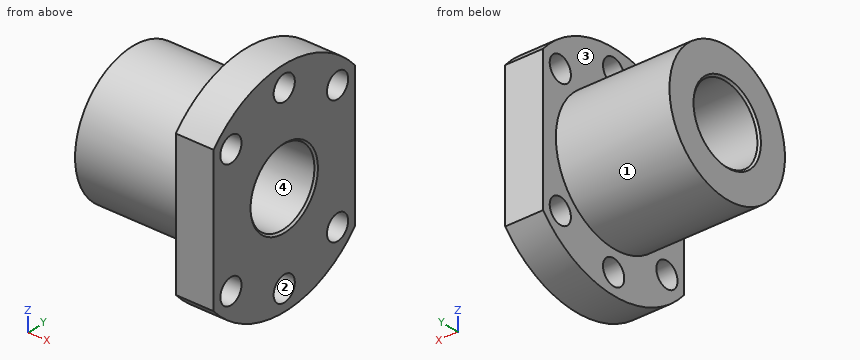
from build123d import *

# Parameters (mm, degrees)
F0_R     = 18
F1_DEPTH = 30
F3_DEPTH = 10
F4_R     = 10
F5_DEPTH = 40.001
F6_SIZE  = 0.5
F8_D     = 6.6


with BuildPart() as f1:
    # F0 (on Right) → F1 (new body)
    with BuildSketch(Plane.YZ):
        Circle(F0_R)
    extrude(amount=-F1_DEPTH)

    # F2 (on face) → F3 (join)
    with BuildSketch(Plane.YZ):
        with BuildLine():
            Line((-22, 18.8944436277), (-22, -18.8944436277))
            ThreePointArc((-22, -18.8944436277), (0, -29), (22, -18.8944436277))
            Line((22, -18.8944436277), (22, 18.8944436277))
            ThreePointArc((22, 18.8944436277), (0, 29), (-22, 18.8944436277))
        make_face()
    extrude(amount=F3_DEPTH)

    # F4 (on face) → F5 (cut, through all)
    with BuildSketch(Plane.YZ.offset(10)):
        Circle(F4_R)
    extrude(amount=-F5_DEPTH, mode=Mode.SUBTRACT)

    # F6
    f6_edges = [f1.edges().sort_by_distance(p)[0] for p in [
        (10, -10, 0),
        (-30, -10, 0),
    ]]
    chamfer(f6_edges, length=F6_SIZE)

    # F8 (through all)
    with Locations(Plane.YZ.offset(10)):
        with Locations((0, 23.5), (16.617, 16.617), (16.617, -16.617), (0, -23.5), (-16.617, -16.617), (-16.617, 16.617)):
            Hole(F8_D / 2)


solid = f1.part
Verification items for the finished model (mm, model axes). Face numbers are marked on the shaded views. Coordinates: 2 decimals unless noted, no trailing zeros. Write each loop counter-clockwise with the first axis right and the second up, starting at its lowest first coordinate (ties: lowest second). Pieces come first, ordered by that corner, then holes. Notation, with made-up numbers: M -35.75,67 L 19.25,67 A34 cw 19.25,100 Z; hole C -31,13.25 d1. An arc over 180 degrees is marked long. Use a Markdown table: item, result.
Q1. Sectioned sample at C-C, the plane x = -17.5. Record the boundary of the cut face in (y, z), plus the area to 3 significant figures.
Reply:
| item | result |
|---|---|
| outline | C 0,0 d36; hole C 0,0 d20 |
| area | 704 mm² |
Q2. Sectioned sample at D-D, the plane y = 17. Record the boundary of the cut face in (x, z), plus the area to 3 significant figures.
Reply:
| item | result |
|---|---|
| outline | M -30,-5.92 L 0,-5.92 L 0,-13.34 L 10,-13.34 L 10,13.34 L 0,13.34 L 0,5.92 L -30,5.92 Z; M 0,-23.49 L 10,-23.49 L 10,-19.89 L 0,-19.89 Z; M 0,19.89 L 10,19.89 L 10,23.49 L 0,23.49 Z |
| area | 694 mm² |
Q3. Draft check along Y on the marked faces 1, 2, 3 and 4. Enter one of: +Y half, -Y half, draft (parallel to the pull), parting line (faces both ways), or undercut.
Reply:
| item | result |
|---|---|
| face 1 | parting line |
| face 2 | undercut |
| face 3 | draft |
| face 4 | undercut |
Q4. Thickness scan on line 1 (Z direction, x = -17.5, y = 0); line 2 (Z direction, x = -21, y = -2.5); line 3 (Y direction, x = 3, z = -23). Record the ranges inside material, lowest first.
Reply:
| item | result |
|---|---|
| line 1 | z = -18 to -10, 10 to 18 |
| line 2 | z = -17.83 to -9.68, 9.68 to 17.83 |
| line 3 | y = -17.66 to -3.26, 3.26 to 17.66 |
Q5. Go/stop test with flat-tipped pins: P1, Ø8.5, axis at y = 0, z = 23.5, coming from the -X side; P2, Ø3, axis at y = -8.5, z = 1.5, coming from the +X side; P3, Ø6, axis at x = -5, z = 14.5, coming from the +Y side. Record where each tip stops, or that it passes through.
Reply:
| item | result |
|---|---|
| P1 | stops at x = 0 |
| P2 | stops at x = 9.63 |
| P3 | stops at y = 13.85 |
Q6. Sectioned sample at A-A, the plane z = 0. Record the boundary of the cut face in (x, y).
Reply:
| item | result |
|---|---|
| outline | M -30,-18 L 0,-18 L 0,-22 L 10,-22 L 10,-10.5 L 9.5,-10 L -29.5,-10 L -30,-10.5 Z; M -30,10.5 L -29.5,10 L 9.5,10 L 10,10.5 L 10,22 L 0,22 L 0,18 L -30,18 Z |
Q7. Sectioned sample at B-B, the plane y = 0. Record the boundary of the cut face in (x, z).
Reply:
| item | result |
|---|---|
| outline | M -30,-18 L 0,-18 L 0,-20.2 L 10,-20.2 L 10,-10.5 L 9.5,-10 L -29.5,-10 L -30,-10.5 Z; M -30,10.5 L -29.5,10 L 9.5,10 L 10,10.5 L 10,20.2 L 0,20.2 L 0,18 L -30,18 Z; M 0,-29 L 10,-29 L 10,-26.8 L 0,-26.8 Z; M 0,26.8 L 10,26.8 L 10,29 L 0,29 Z |
